from build123d import *

# Parameters (mm, degrees)
EXTRUDE_1_DEPTH            = 30
SKETCH_2_R                 = 4.025
EXTRUDE_2_DEPTH            = 8.5
CHAMFER_1_SIZE             = 0.6
CUT_EXTRUDE_1_DEPTH        = 8
CHAMFER_1_OF_MIRROR_1_SIZE = 0.6
CHAMFER_2_SIZE             = 1.5


with BuildPart() as part:
    # 草图1 → 凸台-拉伸1 (new body)
    with BuildSketch(Plane.XY):
        Polygon((5.773502692, 0), (2.886751346, 5), (-2.886751346, 5), (-5.773502692, 0), (-2.886751346, -5), (2.886751346, -5), align=None)
    extrude(amount=EXTRUDE_1_DEPTH)

    # 草图2 → 凸台-拉伸2 (add)
    with BuildSketch(Plane.XY.offset(30)):
        Circle(SKETCH_2_R)
    extrude_2 = extrude(amount=EXTRUDE_2_DEPTH)

    # 倒角1
    chamfer_1_edges = [part.edges().sort_by_distance(p)[0] for p in [
        (-4.025, 0, 38.5),
    ]]
    chamfer(chamfer_1_edges, length=CHAMFER_1_SIZE)

    # 草图3 → 切除-拉伸1 (cut)
    with BuildSketch(Plane.XY.offset(38.5)):
        with BuildLine():
            Line((-1.140175425, 1.05), (1.140175425, 1.05))
            ThreePointArc((1.140175425, 1.05), (0, -1.55), (-1.140175425, 1.05))
        make_face()
    cut_extrude_1 = extrude(amount=-CUT_EXTRUDE_1_DEPTH, mode=Mode.SUBTRACT)

    # 镜向1: 凸台-拉伸2, 切除-拉伸1 across plane
    add(extrude_2.mirror(Plane.XY.offset(15)))
    add(cut_extrude_1.mirror(Plane.XY.offset(15)), mode=Mode.SUBTRACT)

    # 倒角1 of 镜向1
    chamfer_1_of_mirror_1_edges = [part.edges().sort_by_distance(p)[0] for p in [
        (-4.025, 0, -8.5),
    ]]
    chamfer(chamfer_1_of_mirror_1_edges, length=CHAMFER_1_OF_MIRROR_1_SIZE)

    # 倒角2
    # the kernel refuses this chamfer: 1.5 mm, written as the material it takes off along each edge
    with BuildSketch(Plane(origin=(6.744275828, 5, 30), x_dir=(0, 0.02749587661058619, -0.9996219169112968), z_dir=(-1, 0, 0))) as chamfer_2_piece_1_section:
        Polygon((CHAMFER_2_SIZE * 0.999621916911, CHAMFER_2_SIZE * 0.0274958766106), (-CHAMFER_2_SIZE * 0.0274958766106, CHAMFER_2_SIZE * 0.999621916911), (0, 0), align=None)
    chamfer_2_piece_1 = extrude(amount=13.488551656, mode=Mode.PRIVATE)
    chamfer_2_piece_1 = chamfer_2_piece_1 - Plane(origin=(0, 0, 29.496283427), x_dir=(1, 0, 0), z_dir=(0, 0, -1)) * Cylinder(4.025, 33, mode=Mode.PRIVATE)
    add(chamfer_2_piece_1, mode=Mode.SUBTRACT)
    with BuildSketch(Plane(origin=(-0.957989105, 8.340714197, 30), x_dir=(-0.02381212764409015, 0.013747938305292993, -0.9996219169112968), z_dir=(-0.49999999999999506, -0.8660254037844416, 0))) as chamfer_2_piece_2_section:
        Polygon((CHAMFER_2_SIZE * 0.999621916911, CHAMFER_2_SIZE * 0.0274958766106), (-CHAMFER_2_SIZE * 0.0274958766106, CHAMFER_2_SIZE * 0.999621916911), (0, 0), align=None)
    chamfer_2_piece_2 = extrude(amount=13.488551656, mode=Mode.PRIVATE)
    chamfer_2_piece_2 = chamfer_2_piece_2 - Plane(origin=(0, 0, 29.496283427), x_dir=(1, 0, 0), z_dir=(0, 0, -1)) * Cylinder(4.025, 33, mode=Mode.PRIVATE)
    add(chamfer_2_piece_2, mode=Mode.SUBTRACT)
    with BuildSketch(Plane(origin=(-7.702264933, 3.340714197, 30), x_dir=(-0.023812127644089943, -0.013747938305293316, -0.9996219169112968), z_dir=(0.5000000000000071, -0.8660254037844346, 0))) as chamfer_2_piece_3_section:
        Polygon((CHAMFER_2_SIZE * 0.999621916911, CHAMFER_2_SIZE * 0.0274958766106), (-CHAMFER_2_SIZE * 0.0274958766106, CHAMFER_2_SIZE * 0.999621916911), (0, 0), align=None)
    chamfer_2_piece_3 = extrude(amount=13.488551656, mode=Mode.PRIVATE)
    chamfer_2_piece_3 = chamfer_2_piece_3 - Plane(origin=(0, 0, 29.496283427), x_dir=(1, 0, 0), z_dir=(0, 0, -1)) * Cylinder(4.025, 33, mode=Mode.PRIVATE)
    add(chamfer_2_piece_3, mode=Mode.SUBTRACT)
    with BuildSketch(Plane(origin=(-6.744275828, -5, 30), x_dir=(0, -0.02749587661058619, -0.9996219169112968), z_dir=(1, 0, 0))) as chamfer_2_piece_4_section:
        Polygon((CHAMFER_2_SIZE * 0.999621916911, CHAMFER_2_SIZE * 0.0274958766106), (-CHAMFER_2_SIZE * 0.0274958766106, CHAMFER_2_SIZE * 0.999621916911), (0, 0), align=None)
    chamfer_2_piece_4 = extrude(amount=13.488551656, mode=Mode.PRIVATE)
    chamfer_2_piece_4 = chamfer_2_piece_4 - Plane(origin=(0, 0, 29.496283427), x_dir=(1, 0, 0), z_dir=(0, 0, -1)) * Cylinder(4.025, 33, mode=Mode.PRIVATE)
    add(chamfer_2_piece_4, mode=Mode.SUBTRACT)
    with BuildSketch(Plane(origin=(0.957989105, -8.340714197, 30), x_dir=(0.02381212764409026, -0.013747938305293058, -0.9996219169112968), z_dir=(0.49999999999999506, 0.8660254037844416, 0))) as chamfer_2_piece_5_section:
        Polygon((CHAMFER_2_SIZE * 0.999621916911, CHAMFER_2_SIZE * 0.0274958766106), (-CHAMFER_2_SIZE * 0.0274958766106, CHAMFER_2_SIZE * 0.999621916911), (0, 0), align=None)
    chamfer_2_piece_5 = extrude(amount=13.488551656, mode=Mode.PRIVATE)
    chamfer_2_piece_5 = chamfer_2_piece_5 - Plane(origin=(0, 0, 29.496283427), x_dir=(1, 0, 0), z_dir=(0, 0, -1)) * Cylinder(4.025, 33, mode=Mode.PRIVATE)
    add(chamfer_2_piece_5, mode=Mode.SUBTRACT)
    with BuildSketch(Plane(origin=(-6.744275828, -5, 0), x_dir=(-1.0610740769848241e-14, 0.9996219169112969, -0.027495876610586372), z_dir=(1, 0, 0))) as chamfer_2_piece_6_section:
        Polygon((CHAMFER_2_SIZE * 0.999621916911, CHAMFER_2_SIZE * 0.0274958766106), (-CHAMFER_2_SIZE * 0.0274958766106, CHAMFER_2_SIZE * 0.999621916911), (0, 0), align=None)
    chamfer_2_piece_6 = extrude(amount=13.488551656, mode=Mode.PRIVATE)
    chamfer_2_piece_6 = chamfer_2_piece_6 - Plane(origin=(0, 0, 0.503716575), x_dir=(1, 0, 0), z_dir=(0, 0, 1)) * Cylinder(4.025, 33, mode=Mode.PRIVATE)
    add(chamfer_2_piece_6, mode=Mode.SUBTRACT)
    with BuildSketch(Plane(origin=(-7.702264933, 3.340714197, 0), x_dir=(0.8656979742248763, 0.49981095845565543, -0.027495876610586372), z_dir=(0.5000000000000071, -0.8660254037844346, 0))) as chamfer_2_piece_7_section:
        Polygon((CHAMFER_2_SIZE * 0.999621916911, CHAMFER_2_SIZE * 0.0274958766106), (-CHAMFER_2_SIZE * 0.0274958766106, CHAMFER_2_SIZE * 0.999621916911), (0, 0), align=None)
    chamfer_2_piece_7 = extrude(amount=13.488551656, mode=Mode.PRIVATE)
    chamfer_2_piece_7 = chamfer_2_piece_7 - Plane(origin=(0, 0, 0.503716575), x_dir=(1, 0, 0), z_dir=(0, 0, 1)) * Cylinder(4.025, 33, mode=Mode.PRIVATE)
    add(chamfer_2_piece_7, mode=Mode.SUBTRACT)
    with BuildSketch(Plane(origin=(-0.957989105, 8.340714197, 0), x_dir=(0.8656979742248831, -0.4998109584556434, -0.027495876610586365), z_dir=(-0.49999999999999506, -0.8660254037844416, 0))) as chamfer_2_piece_8_section:
        Polygon((CHAMFER_2_SIZE * 0.999621916911, CHAMFER_2_SIZE * 0.0274958766106), (-CHAMFER_2_SIZE * 0.0274958766106, CHAMFER_2_SIZE * 0.999621916911), (0, 0), align=None)
    chamfer_2_piece_8 = extrude(amount=13.488551656, mode=Mode.PRIVATE)
    chamfer_2_piece_8 = chamfer_2_piece_8 - Plane(origin=(0, 0, 0.503716575), x_dir=(1, 0, 0), z_dir=(0, 0, 1)) * Cylinder(4.025, 33, mode=Mode.PRIVATE)
    add(chamfer_2_piece_8, mode=Mode.SUBTRACT)
    with BuildSketch(Plane(origin=(6.744275828, 5, 0), x_dir=(3.2293558864755513e-15, -0.9996219169112969, -0.027495876610586372), z_dir=(-1, 0, 0))) as chamfer_2_piece_9_section:
        Polygon((CHAMFER_2_SIZE * 0.999621916911, CHAMFER_2_SIZE * 0.0274958766106), (-CHAMFER_2_SIZE * 0.0274958766106, CHAMFER_2_SIZE * 0.999621916911), (0, 0), align=None)
    chamfer_2_piece_9 = extrude(amount=13.488551656, mode=Mode.PRIVATE)
    chamfer_2_piece_9 = chamfer_2_piece_9 - Plane(origin=(0, 0, 0.503716575), x_dir=(1, 0, 0), z_dir=(0, 0, 1)) * Cylinder(4.025, 33, mode=Mode.PRIVATE)
    add(chamfer_2_piece_9, mode=Mode.SUBTRACT)
    with BuildSketch(Plane(origin=(7.702264933, -3.340714197, 0), x_dir=(-0.8656979742248797, -0.49981095845564943, -0.027495876610586372), z_dir=(-0.5000000000000011, 0.866025403784438, 0))) as chamfer_2_piece_10_section:
        Polygon((CHAMFER_2_SIZE * 0.999621916911, CHAMFER_2_SIZE * 0.0274958766106), (-CHAMFER_2_SIZE * 0.0274958766106, CHAMFER_2_SIZE * 0.999621916911), (0, 0), align=None)
    chamfer_2_piece_10 = extrude(amount=13.488551656, mode=Mode.PRIVATE)
    chamfer_2_piece_10 = chamfer_2_piece_10 - Plane(origin=(0, 0, 0.503716574), x_dir=(1, 0, 0), z_dir=(0, 0, 1)) * Cylinder(4.025, 33, mode=Mode.PRIVATE)
    add(chamfer_2_piece_10, mode=Mode.SUBTRACT)
    with BuildSketch(Plane(origin=(0.957989105, -8.340714197, 0), x_dir=(-0.8656979742248831, 0.4998109584556434, -0.02749587661058637), z_dir=(0.49999999999999506, 0.8660254037844416, 0))) as chamfer_2_piece_11_section:
        Polygon((CHAMFER_2_SIZE * 0.999621916911, CHAMFER_2_SIZE * 0.0274958766106), (-CHAMFER_2_SIZE * 0.0274958766106, CHAMFER_2_SIZE * 0.999621916911), (0, 0), align=None)
    chamfer_2_piece_11 = extrude(amount=13.488551656, mode=Mode.PRIVATE)
    chamfer_2_piece_11 = chamfer_2_piece_11 - Plane(origin=(0, 0, 0.503716575), x_dir=(1, 0, 0), z_dir=(0, 0, 1)) * Cylinder(4.025, 33, mode=Mode.PRIVATE)
    add(chamfer_2_piece_11, mode=Mode.SUBTRACT)
    with BuildSketch(Plane(origin=(7.702264933, -3.340714197, 30), x_dir=(0.02381212764409016, 0.013747938305293224, -0.9996219169112968), z_dir=(-0.5000000000000011, 0.866025403784438, 0))) as chamfer_2_piece_12_section:
        Polygon((CHAMFER_2_SIZE * 0.999621916911, CHAMFER_2_SIZE * 0.0274958766106), (-CHAMFER_2_SIZE * 0.0274958766106, CHAMFER_2_SIZE * 0.999621916911), (0, 0), align=None)
    chamfer_2_piece_12 = extrude(amount=13.488551656, mode=Mode.PRIVATE)
    chamfer_2_piece_12 = chamfer_2_piece_12 - Plane(origin=(0, 0, 29.496283426), x_dir=(1, 0, 0), z_dir=(0, 0, -1)) * Cylinder(4.025, 33, mode=Mode.PRIVATE)
    add(chamfer_2_piece_12, mode=Mode.SUBTRACT)


solid = part.part
CAD build for the part. Positions are in the model's coordinates, mm. A direction names the side the tool comes from. Round coordinates to 2 decimals unless told otherwise and drop trailing zeros. Write each loop counter-clockwise with the first axis right and the second up, starting at its lowest first coordinate (ties: lowest second). Pieces come first, ordered by that corner, then holes.
(1) Drop flat-ended pins along their axis: P1, Ø1.5, axis at x = -4, z = 19, coming from the +Y side; P2, Ø1.9, axis at x = 0, y = 0, coming from the -Z side; P3, Ø1.5, axis at y = -3, z = 28, coming from the +X side. Give the stop position or say it passes through.
(2) Slice it at B-B, the plane z = 21.5. Write the cut outline in (x, y).
(3) 3-axis set-ups, long thin cutter, end or side, ignore diameter. For faces 1 (the face through (3.84, 1.21, -3.57)), 2 (the face through (4.35, 2.465, 14.811)), 3 (the face through (3.84, -1.21, 33.57)): which of +Z, -Z, +X, -X, +Y, -Y reach the whole face in a straight line?
(4) Slice it at C-C, the plane y = -4.5. Write the cut outline in (x, z).
(5) Mould opens along Y. For faces 4 (the face through (0, 0, -0.5)), 5 (the face through (0, 5, 15)), 6 (the face through (-3.854, -2.179, 29.073)) say: pulls with the +Y half, pulls with the -Y half, needs draft (parallel to the pull), parting line crosses it, or undercut.
(6) Probe line 1 along Y through (x, z) = (0, -4.75) (3 decimals); line 2 along X through (y, z) = (0, -5.75) (3 decimals); line 3 along Z through (x, y) = (-1, -4). List the from-to ranges inside material, lowest first.
(7) Slice it at A-A, the plane x = 0. Write the cut outline in (y, z) (3 decimals), and give its area (3 significant figures).
(8) Slice it at D-D, the plane z = 31.5. Write the cut outline in (x, y) (3 decimals).
From the geometry:
1. P1: stops at y = 4.37
1. P2: stops at z = -0.5
1. P3: stops at x = 4.47
2. outline: (-5.77, 0) - (-2.89, -5) - (2.89, -5) - (5.77, 0) - (2.89, 5) - (-2.89, 5) - close
3. face 1: -Z
3. face 2: +Z, -Z, +X, +Y
3. face 3: +Z
4. outline: (-3.18, 1.5) - (-2.6, 1) - (2.6, 1) - (3.18, 1.5) - (3.18, 28.5) - (2.6, 29) - (-2.6, 29) - (-3.18, 28.5) - close
5. face 4: undercut
5. face 5: pulls with the +Y half
5. face 6: pulls with the -Y half
6. line 1: y = -4.025 to -1.55, 1.05 to 4.025
6. line 2: x = -4.025 to -1.55, 1.55 to 4.025
6. line 3: z = 0.5 to 29.5
7. outline: (-5, 1.5) - (-4.025, 0.525) - (-4.025, -7.9) - (-3.425, -8.5) - (-1.55, -8.5) - (-1.55, -0.5) - (1.05, -0.5) - (1.05, -8.5) - (3.425, -8.5) - (4.025, -7.9) - (4.025, 0.525) - (5, 1.5) - (5, 28.5) - (4.025, 29.475) - (4.025, 37.9) - (3.425, 38.5) - (1.05, 38.5) - (1.05, 30.5) - (-1.55, 30.5) - (-1.55, 38.5) - (-3.425, 38.5) - (-4.025, 37.9) - (-4.025, 29.475) - (-5, 28.5) - close
7. area: 391 mm2
8. outline: circle Ø8.05 at (0, 0); hole (-1.14, 1.05) arc R1.55 ccw (long way) to (1.14, 1.05) - close
